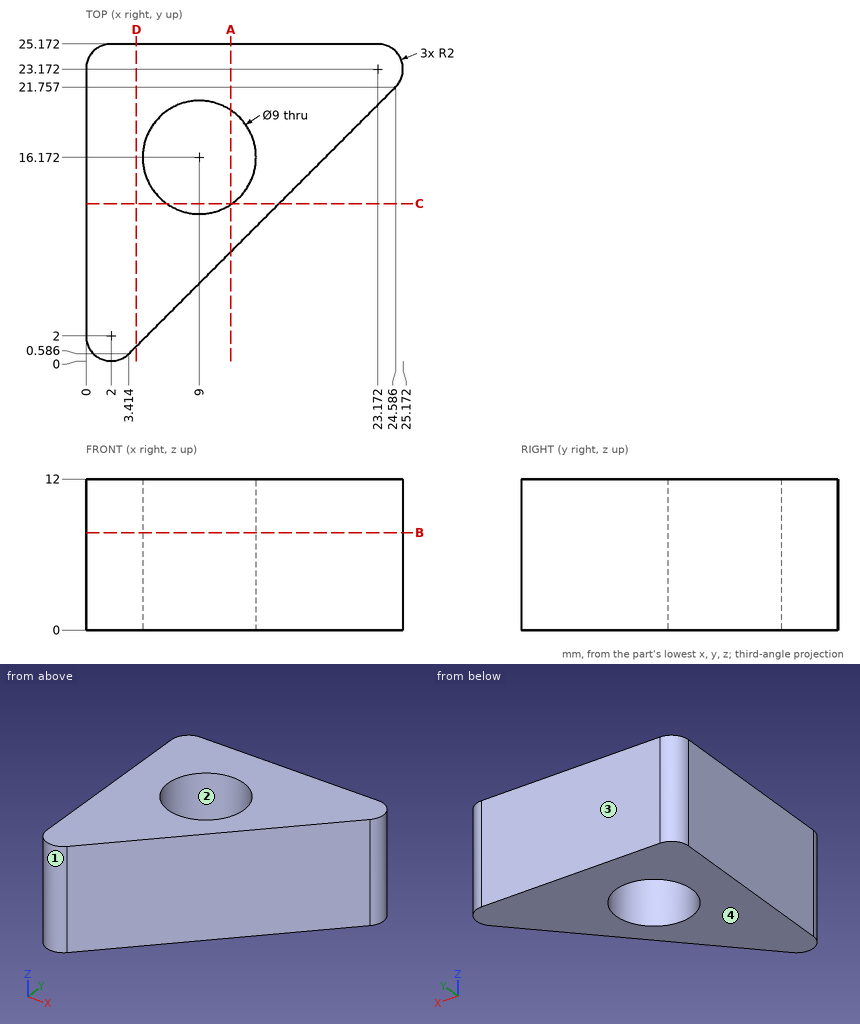
For this review, use the dimensioned drawing (mm, ordinates from the lowest corner) and the shaded views. Coordinates: 2 decimals unless noted, no trailing zeros. Order: outer loops, then holes, each group sorted by start corner. A loop starts at its lowest first (then second) coordinate and runs counter-clockwise, first axis right, second up. Notation, with made-up numbers: (23, 52) - (68, 52) arc R20 cw to (68, 87) - close; hole circle Ø6 at (81.5, -2.5). An arc over 180 degrees is marked (long way). Answer as a JSON object with one key per item and string values. Group by question number.
1. We need section A-A on x = 11.5. State the section outline as (y, z) points.
2. The part is to be moulded in two halves that separate along Y. For the marked faces 1, 2, 3 and 4, say which applies: pulls with the +Y half, pulls with the -Y half, needs draft (parallel to the pull), parting line crosses it, or undercut.
3. Clearance check with flat-ended pins moving along their axes: P1, Ø10.5, axis at x = 9, y = 16.17, coming from the +Z side; P2, Ø2, axis at y = 20.5, z = 7.5, coming from the +X side. State where each tip first meets the part, or that it passes through.
4. We need section C-C on y = 12.5. State the section outline as (x, z) points.
5. For probe 1 along Y at (x, z) = (6.25, 8.5) (1 decimal); probe 2 along Y at (x, z) = (9, 6.5); probe 3 along X at (y, z) = (15.75, 6.75), list the stretches that pass through material, from the lowest coordinate up.
6. We need section B-B on z = 7.75. State the section outline as (x, y) points (1 decimal).
7. We need section D-D on x = 4. State the section outline as (y, z) points, then the cut area to 3 significant figures.
Final values:
{
 "1": {"outline": "(8.67, 0) - (12.43, 0) - (12.43, 12) - (8.67, 12) - close; (19.91, 0) - (25.17, 0) - (25.17, 12) - (19.91, 12) - close"},
 "2": {"face 1": "pulls with the -Y half", "face 2": "undercut", "face 3": "pulls with the +Y half", "face 4": "needs draft"},
 "3": {"P1": "z = 12", "P2": "x = 24.33"},
 "4": {"outline": "(0, 0) - (6.4, 0) - (6.4, 12) - (0, 12) - close; (11.6, 0) - (15.33, 0) - (15.33, 12) - (11.6, 12) - close"},
 "5": {"probe 1": "3.4 to 12.6, 19.7 to 25.2", "probe 2": "6.17 to 11.67, 20.67 to 25.17", "probe 3": "0 to 4.52, 13.48 to 18.58"},
 "6": {"outline": "(0, 2) arc R2 ccw to (3.4, 0.6) - (24.6, 21.8) arc R2 ccw to (23.2, 25.2) - (2, 25.2) arc R2 ccw to (0, 23.2) - close; hole circle Ø9 at (9, 16.2)"},
 "7": {"outline": "(1.17, 0) - (25.17, 0) - (25.17, 12) - (1.17, 12) - close", "area": "288 mm²"}
}
